The listing builds one solid part. Answer for the finished solid, in the listing's coordinates (mm). A direction names the side the tool comes from. Round coordinates to 2 decimals unless told otherwise and drop trailing zeros. Order: outer loops, then holes, each group sorted by start corner. A loop starts at its lowest first (then second) coordinate and runs counter-clockwise, first axis right, second up. Notation, with made-up numbers: (-36, 59) - (-3, 59) arc R21 cw to (-3, 95) - close; hole circle Ø10 at (74, -26.5). An arc over 180 degrees is marked (long way). Use CSV: the item, a comma, the result in double quotes. Start each with the question number.
Item 1: Flat-ended cylindrical pins translate along their axes: P1, Ø5.5, axis at x = 0, z = 63.5, coming from the -Y side; P2, Ø1, axis at y = -2, z = 32, coming from the -X side. Find the tip coordinate at first contact, or state that the pin passes through.
Item 2: Determine the mould class of faces 1 (the flat face through (-12.6, -1.5, 90.2)), 2 (the flat face through (-12.68, -1.5, 30.92)), 3 (the cylindrical face through (3.805, -1.503, 1.198)), 4 (the cylindrical face through (-15.873, -1.503, 63.737)) for opening direction Z: +Z half, -Z half, draft (parallel to the pull), parting line (faces both ways), or undercut.
Item 3: Find section D-D, the plane z = 81.5. Give the vertices of the cut face in (x, y) (3 decimals), plus the area to 3 significant figures.
Item 4: Find section B-B, the plane y = -2.2. Count the separate pieces of the cut face and the enclosed holes in it, plus the area to 3 significant figures.
Item 5: Straight lines are drawn through the part: line 1 along Z through (x, y) = (0, -2.4) (3 decimals); line 2 along Z through (x, y) = (40.5, -2.2); line 3 along X through (y, z) = (-2.4, 116). For each, find the intervals that lie inside material, in ascending order. Write a range as [from, to].
Item 6: Find section A-A, the plane x = 48. Give the vertices of the cut face in (y, z).
Item 7: Find section C-C, the plane x = 12. Give the vertices of the cut face in (y, z).
Item 8: For faces 5 (the flat face through (12.925, -1.503, 39.362)), 6 (the cylindrical face through (-6.46, -1.5, -7)), determine the directions among +Z, -Z, +X, -X, +Y, -Y from which every point of the face is accessible in a straight line to the end or side of a thin tool.
```python
from build123d import *

# Parameters (mm, degrees)
F0_R     = 3.175
F0_R_2   = 1.5875
F0_R_3   = 4.729967
F0_R_4   = 3.988899
F0_R_5   = 4.752778
F1_DEPTH = 3.048


with BuildPart() as f1:
    # F0 (on Front) → F1 (new body)
    with BuildSketch(Plane.XZ):
        with BuildLine():
            ThreePointArc((-9.525, 114.3), (0, 104.775), (9.525, 114.3))
            ThreePointArc((9.525, 114.3), (0, 123.825), (-9.525, 114.3))
        make_face()
        with Locations((0, 114.3)):
            Circle(F0_R, mode=Mode.SUBTRACT)
        with BuildLine():
            Line((15.386538, 67.407692), (9.525, 114.3))
            ThreePointArc((9.525, 114.3), (0, 104.775), (-9.525, 114.3))
            Line((-9.525, 114.3), (-15.747457, 65.508289))
            ThreePointArc((-15.747457, 65.508289), (-0.966695, 79.34554), (15.386538, 67.407692))
        make_face()
        with Locations((-4.299854, 100.0252)):
            Circle(F0_R_2, mode=Mode.SUBTRACT)
        with BuildLine():
            Line((15.875, 63.5), (15.386538, 67.407692))
            ThreePointArc((15.386538, 67.407692), (-0.966695, 79.34554), (-15.747457, 65.508289))
            ThreePointArc((-15.747457, 65.508289), (-15.873588, 63.711757), (-15.795426, 61.9125))
            ThreePointArc((-15.795426, 61.9125), (-0.211757, 47.626412), (15.747457, 61.491711))
            ThreePointArc((15.747457, 61.491711), (15.843082, 62.493832), (15.875, 63.5))
        make_face()
        with Locations((0, 63.5)):
            Circle(F0_R_3, mode=Mode.SUBTRACT)
        with BuildLine():
            ThreePointArc((15.875, 63.5), (15.752411, 65.469051), (15.386538, 67.407692))
            Line((15.386538, 67.407692), (15.875, 63.5))
        make_face()
        with BuildLine():
            ThreePointArc((15.747457, 61.491711), (-0.211757, 47.626412), (-15.795426, 61.9125))
            Line((-15.795426, 61.9125), (-9.477255, -0.9525))
            ThreePointArc((-9.477255, -0.9525), (-0.476848, 9.513056), (9.525, 0))
            ThreePointArc((9.525, 0), (6.970557, -6.491299), (0.677344, -9.500886))
            Line((0.677344, -9.500886), (44.732405, -7.932475))
            ThreePointArc((44.732405, -7.932475), (36.5125, 0), (44.732405, 7.932475))
            Line((44.732405, 7.932475), (17.784333, 8.891857))
            ThreePointArc((17.784333, 8.891857), (12.008013, 11.68998), (10.180863, 17.842775))
            Line((10.180863, 17.842775), (15.747457, 61.491711))
        make_face()
        with BuildLine():
            ThreePointArc((9.525, 0), (-0.476848, 9.513056), (-9.477255, -0.9525))
            ThreePointArc((-9.477255, -0.9525), (-6.389564, -7.063929), (0, -9.525))
            Line((0, -9.525), (0.677344, -9.500886))
            ThreePointArc((0.677344, -9.500886), (6.970557, -6.491299), (9.525, 0))
        make_face()
        Circle(F0_R_4, mode=Mode.SUBTRACT)
        with BuildLine():
            Line((0.677344, -9.500886), (0, -9.525))
            ThreePointArc((0, -9.525), (0.338886, -9.51897), (0.677344, -9.500886))
        make_face()
        with BuildLine():
            ThreePointArc((52.3875, 0), (50.161633, 5.51191), (44.732405, 7.932475))
            ThreePointArc((44.732405, 7.932475), (36.5125, 0), (44.732405, -7.932475))
            ThreePointArc((44.732405, -7.932475), (50.161633, -5.51191), (52.3875, 0))
        make_face()
        with Locations((44.45, 0)):
            Circle(F0_R_5, mode=Mode.SUBTRACT)
    extrude(amount=F1_DEPTH)


solid = f1.part
```
Worked out:
1,P1,"passes through"
1,P2,"stops at x = -12.84"
2,face 1,"+Z half"
2,face 2,"-Z half"
2,face 3,"undercut"
2,face 4,"parting line"
3,outline,"(-13.708, -3.048) - (13.625, -3.048) - (13.625, 0) - (-13.708, 0) - close"
3,area,"83.3 mm²"
4,separate pieces,"1"
4,enclosed holes,"5"
4,area,"3,660 mm²"
5,line 1,"z = [-9.525, -3.989], [3.989, 58.77], [68.23, 111.125], [117.475, 123.825]"
5,line 2,"z = [-8.08, -2.64], [2.64, 8.08]"
5,line 3,"x = [-9.37, -2.68], [2.68, 9.37]"
6,outline,"(-3.05, -7.1) - (0, -7.1) - (0, -3.16) - (-3.05, -3.16) - close; (-3.05, 3.16) - (0, 3.16) - (0, 7.1) - (-3.05, 7.1) - close"
7,outline,"(-3.05, -9.1) - (0, -9.1) - (0, 11.7) - (-3.05, 11.7) - close; (-3.05, 32.11) - (0, 32.11) - (0, 94.5) - (-3.05, 94.5) - close"
8,face 5,"+X, +Y, -Y"
8,face 6,"-Z, -X, +Y, -Y"
